Geometry check sheet. Reference: the model listing, model coordinates, mm. Coordinates: 2 decimals unless noted, no trailing zeros. Loops run counter-clockwise (first coordinate to the right, second up) from the corner with the lowest first, then second, coordinate; pieces in that order, holes last.
from build123d import *

# Parameters (mm, degrees)
F1_DEPTH    = 12
F2_T1_DEPTH = 12
F3_R        = 60


# Not quite as in the source:
# - a fillet or chamfer that OpenCascade refuses, or shapes differently, is made with other operations: its cross-section is extruded or revolved along the edge and cut away or added


with BuildPart() as f1:
    # F0 (on Top) → F1 (new body)
    with BuildSketch(Plane.XY):
        Polygon((132.5, 193), (132.5, 181), (137.5, 181), (142.5, 181), (142.5, 193), (137.5, 193), align=None)
        Polygon((27.3656716418, 193), (25.6641791045, 181), (37.7842070275, 181), (39.4856995648, 193), align=None)
        Polygon((25.6641791045, 181), (19.9925373134, 141), (32.1125652364, 141), (37.7842070275, 181), align=None)
        Polygon((19.9925373134, 141), (18.2910447761, 129), (30.4110726991, 129), (32.1125652364, 141), align=None)
        Polygon((237.2157929725, 181), (242.8874347636, 141), (255.0074626866, 141), (249.3358208955, 181), align=None)
        Polygon((235.5143004352, 193), (237.2157929725, 181), (249.3358208955, 181), (247.6343283582, 193), align=None)
        Polygon((242.8874347636, 141), (244.5889273009, 129), (256.7089552239, 129), (255.0074626866, 141), align=None)
        Polygon((244.5889273009, 129), (251.6784795397, 79), (263.7985074627, 79), (256.7089552239, 129), align=None)
        Polygon((251.6784795397, 79), (253.379972077, 67), (265.5, 67), (263.7985074627, 79), align=None)
        Polygon((132.5, 79), (132.5, 67), (137.5, 67), (142.5, 67), (142.5, 79), (137.5, 79), align=None)
        Polygon((253.379972077, 67), (261.1784795397, 12), (273.2985074627, 12), (265.5, 67), align=None)
        Polygon((261.1784795397, 12), (262.879972077, 0), (275, 0), (273.2985074627, 12), align=None)
        Polygon((13.8215204603, 12), (12.120027923, 0), (62.6201442689, 0), (64.3216368062, 12), align=None)
        Polygon((1.7014925373, 12), (0, 0), (12.120027923, 0), (13.8215204603, 12), align=None)
        Polygon((9.5, 67), (1.7014925373, 12), (13.8215204603, 12), (21.620027923, 67), align=None)
        Polygon((11.2014925373, 79), (9.5, 67), (21.620027923, 67), (23.3215204603, 79), align=None)
        Polygon((18.2910447761, 129), (11.2014925373, 79), (23.3215204603, 79), (30.4110726991, 129), align=None)
        Polygon((132.5, 141), (132.5, 129), (137.5, 129), (142.5, 129), (142.5, 141), (137.5, 141), align=None)
        Polygon((72.1201442689, 67), (64.3216368062, 12), (76.4416647292, 12), (84.2401721919, 67), align=None)
        Polygon((80.911189045, 129), (73.8216368062, 79), (85.9416647292, 79), (93.031216968, 129), align=None)
        Polygon((88.2843233734, 181), (82.6126815823, 141), (94.7327095053, 141), (100.4043512964, 181), align=None)
        Polygon((39.4856995648, 193), (37.7842070275, 181), (88.2843233734, 181), (89.9858159107, 193), align=None)
        Polygon((102.1058438337, 193), (100.4043512964, 181), (132.5, 181), (132.5, 193), align=None)
        Polygon((142.5, 193), (142.5, 181), (174.5956487036, 181), (172.8941561663, 193), align=None)
        Polygon((185.0141840893, 193), (186.7156766266, 181), (237.2157929725, 181), (235.5143004352, 193), align=None)
        Polygon((172.8941561663, 193), (174.5956487036, 181), (186.7156766266, 181), (185.0141840893, 193), align=None)
        Polygon((174.5956487036, 181), (180.2672904947, 141), (192.3873184177, 141), (186.7156766266, 181), align=None)
        Polygon((180.2672904947, 141), (181.968783032, 129), (194.088810955, 129), (192.3873184177, 141), align=None)
        Polygon((181.968783032, 129), (189.0583352708, 79), (201.1783631938, 79), (194.088810955, 129), align=None)
        Polygon((189.0583352708, 79), (190.7598278081, 67), (202.8798557311, 67), (201.1783631938, 79), align=None)
        Polygon((190.7598278081, 67), (198.5583352708, 12), (210.6783631938, 12), (202.8798557311, 67), align=None)
        Polygon((210.6783631938, 12), (212.3798557311, 0), (262.879972077, 0), (261.1784795397, 12), align=None)
        Polygon((198.5583352708, 12), (200.2598278081, 0), (212.3798557311, 0), (210.6783631938, 12), align=None)
        Polygon((142.5, 12), (142.5, 0), (200.2598278081, 0), (198.5583352708, 12), align=None)
        Polygon((132.5, 12), (132.5, 0), (142.5, 0), (142.5, 12), (137.5, 12), align=None)
        Polygon((76.4416647292, 12), (74.7401721919, 0), (132.5, 0), (132.5, 12), align=None)
        Polygon((64.3216368062, 12), (62.6201442689, 0), (74.7401721919, 0), (76.4416647292, 12), align=None)
        Polygon((132.5, 67), (132.5, 12), (137.5, 12), (142.5, 12), (142.5, 67), (137.5, 67), align=None)
        Polygon((132.5, 129), (132.5, 79), (137.5, 79), (142.5, 79), (142.5, 129), (137.5, 129), align=None)
        Polygon((132.5, 181), (132.5, 141), (137.5, 141), (142.5, 141), (142.5, 181), (137.5, 181), align=None)
        Polygon((89.9858159107, 193), (88.2843233734, 181), (100.4043512964, 181), (102.1058438337, 193), align=None)
        Polygon((82.6126815823, 141), (80.911189045, 129), (93.031216968, 129), (94.7327095053, 141), align=None)
        Polygon((73.8216368062, 79), (72.1201442689, 67), (84.2401721919, 67), (85.9416647292, 79), align=None)
    extrude(amount=F1_DEPTH)

    # F2: fillet of radius 60 on 2 edges, made by hand

    # F2_s2 → F2_t1 (join)
    with BuildSketch(Plane.XY):
        with BuildLine():
            ThreePointArc((186.7156872707, 181.0003998584), (225.0552814168, 165.8005010735), (244.5264534747, 129.4434541493))
            Line((244.5264534747, 129.4434541493), (250.4671955698, 130.2857981777))
            ThreePointArc((250.4671955698, 130.2857981777), (246.8116672993, 156.0640430257), (243.1565350676, 181.8423440284))
            Line((243.1565350676, 181.8423440284), (237.2157929725, 187.0001633397))
            ThreePointArc((237.2157929725, 187.0001633397), (211.9657401216, 187.0001633397), (186.8753527454, 186.9984384577))
            Line((186.8753527454, 186.9984384577), (186.7156872707, 181.0003998584))
        make_face()
        with BuildLine():
            ThreePointArc((30.4735465253, 129.4434541493), (49.9447185832, 165.8005010735), (88.2843127293, 181.0003998584))
            Line((88.2843127293, 181.0003998584), (88.1246472546, 186.9984384577))
            ThreePointArc((88.1246472546, 186.9984384577), (63.0342598784, 187.0001633397), (37.7842070275, 187.0001633397))
            Line((37.7842070275, 187.0001633397), (31.8434649324, 181.8423440284))
            ThreePointArc((31.8434649324, 181.8423440284), (28.1883327007, 156.0640430257), (24.5328044302, 130.2857981777))
            Line((24.5328044302, 130.2857981777), (30.4735465253, 129.4434541493))
        make_face()
    extrude(amount=F2_T1_DEPTH)

    # F3
    f3_edges = [f1.edges().sort_by_distance(p)[0] for p in [
        (27.365672, 193, 6),
        (247.634328, 193, 6),
    ]]
    fillet(f3_edges, radius=F3_R)


solid = f1.part
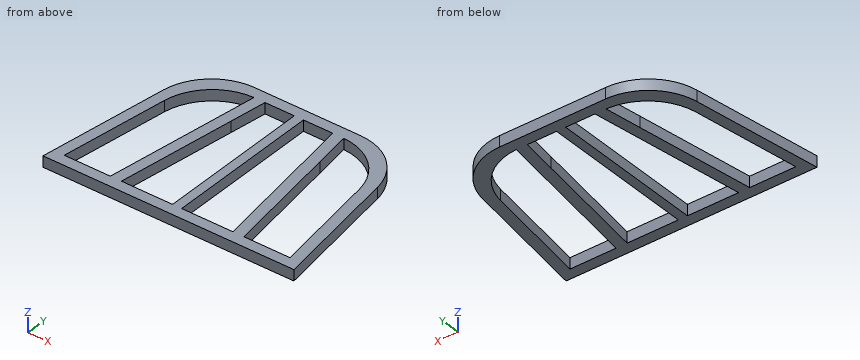
1) Depth check by flat-ended pin: pin 1 (6 mm diameter, centred on x = 38.5, z = 1.5, fed in from +Y); pin 2 (2 mm diameter, centred on y = 49, z = 9, fed in from +X); pin 3 (3 mm diameter, centred on y = 67, z = 4, fed in from +X). Enter the tip coordinate at first touch or a pass-through.
Data:
pin 1: stops at y = 179.47
pin 2: stops at x = 268.19
pin 3: stops at x = 265.71
2) Material ranges on probe 1 along X at (y, z) = (58, 3.25); probe 2 along X at (y, z) = (27.5, 9.75); probe 3 along Y at (x, z) = (111, 10), recorded low to high.
Data:
probe 1: x = 8.22 to 20.34, 70.84 to 82.96, 132.5 to 142.5, 192.04 to 204.16, 254.66 to 266.78
probe 2: x = 3.9 to 16.02, 66.52 to 78.64, 132.5 to 142.5, 196.36 to 208.48, 258.98 to 271.1
probe 3: y = 0 to 12, 181 to 193
3) Section check A-A on x = 177.5. Record the cut outline in (y, z), and give its area (3 significant figures).
Data:
outline: (0, 0) - (12, 0) - (12, 12) - (0, 12) - close; (160.52, 0) - (193, 0) - (193, 12) - (160.52, 12) - close
area: 534 mm2
4) Section check C-C on z = 3.5. Count the separate pieces of the cut face and the enclosed holes in it, and give its area (3 significant figures).
Data:
separate pieces: 1
enclosed holes: 4
area: 15,800 mm2
5) Section check B-B on y = 30.5. Record the cut outline in (x, z).
Data:
outline: (4.32, 0) - (16.44, 0) - (16.44, 12) - (4.32, 12) - close; (66.94, 0) - (79.06, 0) - (79.06, 12) - (66.94, 12) - close; (132.5, 0) - (142.5, 0) - (142.5, 12) - (132.5, 12) - close; (195.94, 0) - (208.06, 0) - (208.06, 12) - (195.94, 12) - close; (258.56, 0) - (270.68, 0) - (270.68, 12) - (258.56, 12) - close
